CAD build for the part. Positions are in the model's coordinates, mm. Round coordinates to 2 decimals unless told otherwise and drop trailing zeros. Loops run counter-clockwise (first coordinate to the right, second up) from the corner with the lowest first, then second, coordinate; pieces in that order, holes last. Notation, with made-up numbers: M 78,18.25 L 126,18.25 A5 ccw 126,23.25 Z; hole C 31.5,31 d4. An arc over 180 degrees is marked long. One line per item, written item: value. Start each with the question number.
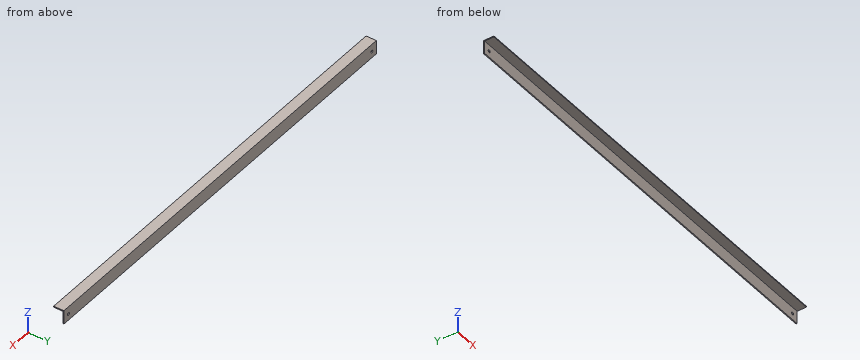
from build123d import *

# Parameters (mm, degrees)
EXTRUDE002_DEPTH = 637
SKETCH016_R      = 2.05
HOLE009_DEPTH    = 1276.481784


with BuildPart() as part:
    # Sketch015 → Extrude002 (new body)
    with BuildSketch(Plane(origin=(0, 0, 0), x_dir=(0, -1, 0), z_dir=(-1, 0, 0))):
        Polygon((-15, 0), (-15, 20), (0, 20), (0, 18.5), (-13.5, 18.5), (-13.5, 0), align=None)
    extrude(amount=-EXTRUDE002_DEPTH)

    # Sketch016 → Hole009 (cut, through all)
    with BuildSketch(Plane.XZ.offset(-13.5)):
        with Locations((9.25, 9.25)):
            Circle(SKETCH016_R)
    hole009 = extrude(amount=-HOLE009_DEPTH, mode=Mode.SUBTRACT)

    # Mirrored005: Hole009 across Sketch016 Axis0
    add(hole009.mirror(Plane(origin=(318.5, 13.5, 18.5), x_dir=(0, -1, 0), z_dir=(1, 0, 0))), mode=Mode.SUBTRACT)


with BuildPart() as part_1:
    # Body007 placement: moved
    add(part.part.moved(Location((1.5, 303.5, 280))))


solid = part_1.part
(1) Flat gauge pins, fed straight in: P1, Ø1, axis at x = 372, z = 292.5, coming from the -Y side; P2, Ø3.5, axis at x = 629.25, z = 289.25, coming from the -Y side; P3, Ø2, axis at x = 284.5, y = 315.5, coming from the -Z side. Where does each tip first touch, or does it go through?
(2) Slice it at C-C, the plane y = 305.75. List the corners of the cut face in (x, z).
(3) Slice it at B-B, the plane z = 283.5. List the corners of the cut face in (x, y), and give its area (4 significant figures).
(4) Probe L1, parallel to X at y = 317.5, z = 289.25; L2, parallel to Z at x = 10.75, y = 317.45; L3, parallel to Y at x = 547, z = 285.5. List the from-to ranges inside material, lowest first.
(5) Slice it at A-A, the plane x = 178.5. List the corners of the cut face in (y, z).
Check result:
1. P1: stops at y = 317
1. P2: passes through
1. P3: stops at z = 298.5
2. outline: M 1.5,298.5 L 638.5,298.5 L 638.5,300 L 1.5,300 Z
3. outline: M 1.5,317 L 638.5,317 L 638.5,318.5 L 1.5,318.5 Z
3. area: 955.5 mm^2
4. L1: x = 1.5 to 8.7, 12.8 to 627.2, 631.3 to 638.5
4. L2: z = 280 to 287.2, 291.3 to 300
4. L3: y = 317 to 318.5
5. outline: M 303.5,298.5 L 317,298.5 L 317,280 L 318.5,280 L 318.5,300 L 303.5,300 Z
